Read the model definition and answer for the solid it produces. Units are mm, in the model's axes. Face numbers are marked on the shaded views. A direction names the side the tool comes from. Round coordinates to 2 decimals unless told otherwise and drop trailing zeros. Order: outer loops, then holes, each group sorted by start corner. A loop starts at its lowest first (then second) coordinate and runs counter-clockwise, first axis right, second up.
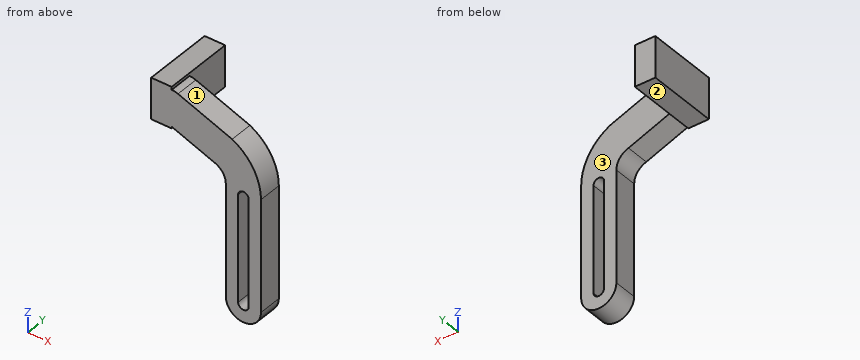
Autodesk Inventor part; units mm, degrees
ref_plane "YZ Plane" through (0, 0, 0) normal (1, 0, 0) x (0, 1, 0)
ref_plane "XZ Plane" through (0, 0, 0) normal (0, 1, 0) x (-1, 0, 0)
ref_plane "XY Plane" through (0, 0, 0) normal (0, 0, 1) x (1, 0, 0)
sketch "Sketch1" plane through (0, 0, 0) normal (0, 1, 0) x (-1, 0, 0)
  line L0 (0, 0) -> (0, 19) construction
  line L1 (-3, 0) -> (-3, 19)
  line L2 (3, 19) -> (3, 0)
  arc A0 (-3, 0) -> (3, 0) centre (0, 0) ccw
  arc A1 (3, 19) -> (-3, 19) centre (0, 19) ccw construction
  line L3 (0, 19) -> (3, 24.1962) construction
  line L4 (2.5981, 17.5) -> (5.5981, 22.6962) construction
  line L5 (0.4019, 25.6962) -> (-2.5981, 20.5) construction
  arc A2 (-2.5981, 20.5) -> (2.5981, 17.5) centre (0, 19) ccw construction
  arc A3 (5.5981, 22.6962) -> (0.4019, 25.6962) centre (3, 24.1962) ccw construction
  line L6 (3, 24.1962) -> (12.2269, 27.738) construction
  line L7 (2.8111, 20.9102) -> (13.302, 24.9373) construction
  line L8 (11.1518, 30.5388) -> (1.9249, 26.9969) construction
  arc A4 (1.9249, 26.9969) -> (1.5, 21.5981) centre (3, 24.1962) ccw construction
  arc A5 (13.302, 24.9373) -> (11.1518, 30.5388) centre (12.2269, 27.738) ccw
  line L9 (12.2269, 27.738) -> (21.2256, 27.8951) construction
  arc A6 (5.0669, 21.7761) -> (3, 19) centre (5.8978, 19) ccw
  line L10 (5.0669, 21.7761) -> (13.302, 24.9373)
  line L11 (1.9249, 26.9969) -> (11.1518, 30.5388)
  arc A7 (1.9249, 26.9969) -> (-3, 19) centre (5.955, 19) ccw
  point P0 (0, 9.5)
  point P1 (1.5, 21.5981)
  point P2 (-2.5981, 20.5)
  point P3 (3, 18.1962)
  point P4 (7.6135, 25.9671)
  point P5 (1.9249, 26.9969)
  point P6 (16.7262, 27.8166)
  dimension "d0" = 6
  dimension "d5" = 25
  dimension "d6" = 150
  dimension "d7" = 6
  dimension "d8" = 12
  dimension "d9" = 12
  dimension "d10" = 111
  dimension "d11" = 200
  dimension "d13" = 9
extrude "Extrusion1" add sketch "Sketch1" along normal mid plane 4
sketch "Sketch2" plane through (0, 2, 0) normal (0, 1, 0) x (1, 0, 0)
  line L0 (0, 0) -> (0, -18.1) construction
  line L1 (-0.9, 0) -> (-0.9, -18.1)
  line L2 (0.9, -18.1) -> (0.9, 0)
  arc A0 (0.9, 0) -> (-0.9, 0) centre (0, 0) ccw
  arc A1 (-0.9, -18.1) -> (0.9, -18.1) centre (0, -18.1) ccw
  point P0 (0, -9.05)
  point P1 (-3, -19)
  point P2 (0, -19)
  dimension "d14" = 1.8
extrude "Extrusion2" cut sketch "Sketch2" against normal through all
sketch "Sketch3" plane through (0, 0, 0) normal (0, 1, 0) x (-1, 0, 0)
  line L0 (-0.9, 0) -> (-0.9, 18.1)
  arc A0 (0.9, 18.1) -> (-0.9, 18.1) centre (0, 18.1) ccw
  line L1 (0.9, 18.1) -> (0.9, 0)
  arc A1 (-0.9, 0) -> (0.9, 0) centre (0, 0) ccw
  arc A2 (-3, 0) -> (3, 0) centre (0, 0) ccw
  line L2 (3, 0) -> (3, 19)
  arc A3 (5.0669, 21.7761) -> (3, 19) centre (5.8978, 19) ccw
  line L3 (5.0669, 21.7761) -> (13.302, 24.9373)
  arc A4 (13.302, 24.9373) -> (11.1518, 30.5388) centre (12.2269, 27.738) ccw
  line L4 (11.1518, 30.5388) -> (1.9249, 26.9969)
  arc A5 (1.9249, 26.9969) -> (-3, 19) centre (5.955, 19) ccw
  line L5 (-3, 19) -> (-3, 0)
  line L6 (15.7269, 24.238) -> (12.2269, 24.238)
  line L7 (12.2269, 24.238) -> (12.2269, 31.238)
  line L8 (12.2269, 31.238) -> (15.7269, 31.238)
  line L9 (15.7269, 31.238) -> (15.7269, 24.238)
  line L10 (13.9769, 24.238) -> (13.9769, 31.238) construction
  line L11 (12.2269, 27.738) -> (15.7269, 27.738) construction
  dimension "d17" = 7
  dimension "d18" = 3.5
extrude "Extrusion3" add sketch "Sketch3" along normal blind 10 and the other way blind 2 contours L7 A4 L3 | L3 A4 L7 L8 L9 L6
sketch "Sketch5" plane through (0, 2, 0) normal (0, 1, 0) x (1, 0, 0)
  point P0 (0, 0)
equation "\"d7\" = d0"
properties part number "_3DPrint"
Q1. A cutting plane is placed at B-B, the plane y = 1. Give the vertices of the cut face in (x, z).
Outcome:
outline: (-15.73, 24.24) - (-12.23, 24.24) - (-12.23, 24.52) - (-5.07, 21.78) arc R2.9 cw to (-3, 19) - (-3, 0) arc R3 ccw to (3, 0) - (3, 19) arc R8.95 ccw to (-1.92, 27) - (-11.15, 30.54) arc R3 ccw to (-12.23, 30.74) - (-12.23, 31.24) - (-15.73, 31.24) - close; hole (-0.9, 0) arc R0.9 ccw to (0.9, 0) - (0.9, 18.1) arc R0.9 ccw to (-0.9, 18.1) - close
Q2. A cutting plane is placed at C-C, the plane x = 0.25. Give the vertices of the cut face in (y, z).
Outcome:
outline: (-2, -2.99) - (2, -2.99) - (2, -0.86) - (-2, -0.86) - close; (-2, 18.96) - (2, 18.96) - (2, 25.46) - (-2, 25.46) - close
Q3. For the marked faces 1, 2 and 3, determine the directions among +Z, -Z, +X, -X, +Y, -Y from which every point of the face is accessible in a straight line to the end or side of a thin tool.
Outcome:
face 1: +Z, +X, +Y, -Y
face 2: -Z, -X, +Y, -Y
face 3: +Z, -Z, +X, +Y
Q4. Straight lines are drawn through the part: probe 1 along X at (y, z) = (-0.25, 8.5); probe 2 along Y at (x, z) = (-9.75, 28); probe 3 along Z at (x, y) = (-14, 2). For each, find the intervals that lie inside material, in ascending order.
Outcome:
probe 1: x = -3 to -0.9, 0.9 to 3
probe 2: y = -2 to 2
probe 3: z = 24.24 to 31.24
Q5. Flat-ended cylindrical pins translate along their axes: pin 1 (7.5 mm diameter, centred on x = -7, z = 6, fed in from +Y); pin 2 (1.8 mm diameter, centred on x = -14.5, y = 5.5, fed in from -Z); pin 3 (1.2 mm diameter, centred on y = 0.5, z = 8.5, fed in from -X); pin 4 (2 mm diameter, centred on x = -3.5, z = 13, fed in from +Y). Find the tip coordinate at first contact, or state that the pin passes through.
Outcome:
pin 1: passes through
pin 2: stops at z = 24.24
pin 3: stops at x = -3
pin 4: stops at y = 2
Q6. A cutting plane is placed at D-D, the plane y = 7.5. Give the vertices of the cut face in (x, z), plus the area to 3 significant figures.
Outcome:
outline: (-15.73, 24.24) - (-12.23, 24.24) - (-12.23, 31.24) - (-15.73, 31.24) - close
area: 24.5 mm2
Q7. A cutting plane is placed at A-A, the plane z = 15. Give the vertices of the cut face in (x, y).
Outcome:
outline: (-3, -2) - (-0.9, -2) - (-0.9, 2) - (-3, 2) - close; (0.9, -2) - (3, -2) - (3, 2) - (0.9, 2) - close
